from build123d import *

# Parameters (mm, degrees)
SKETCH1_W           = 160
SKETCH1_H           = 160
BOSS_EXTRUDE1_DEPTH = 18
SKETCH3_R           = 2
CUT_EXTRUDE1_DEPTH  = 115.560027933
SKETCH4_W           = 10
SKETCH4_H           = 18
BOSS_EXTRUDE3_DEPTH = 160
SKETCH7_R           = 2.75
CUT_EXTRUDE4_DEPTH  = 122.753850042


with BuildPart() as part:
    # Sketch1 → Boss-Extrude1 (new body)
    with BuildSketch(Plane.XY):
        Rectangle(SKETCH1_W, SKETCH1_H)
    extrude(amount=-BOSS_EXTRUDE1_DEPTH)

    # Sketch3 → Cut-Extrude1 (cut, through all)
    with BuildSketch(Plane.XY):
        with Locations((-76.5, 67.5)):
            Circle(SKETCH3_R)
        with Locations((-56.5, 67.5)):
            Circle(SKETCH3_R)
        with Locations((-56.5, 47.5)):
            Circle(SKETCH3_R)
        with Locations((-76.5, 47.5)):
            Circle(SKETCH3_R)
        with Locations((76.5, 67.5)):
            Circle(SKETCH3_R)
        with Locations((76.5, 47.5)):
            Circle(SKETCH3_R)
        with Locations((76.5, -47.5)):
            Circle(SKETCH3_R)
        with Locations((76.5, -67.5)):
            Circle(SKETCH3_R)
        with Locations((56.5, -47.5)):
            Circle(SKETCH3_R)
        with Locations((56.5, -67.5)):
            Circle(SKETCH3_R)
        with Locations((-56.5, -47.5)):
            Circle(SKETCH3_R)
        with Locations((-56.5, -67.5)):
            Circle(SKETCH3_R)
        with Locations((-76.5, -47.5)):
            Circle(SKETCH3_R)
        with Locations((-76.5, -67.5)):
            Circle(SKETCH3_R)
        with Locations((56.5, 67.5)):
            Circle(SKETCH3_R)
        with Locations((56.5, 47.5)):
            Circle(SKETCH3_R)
    extrude(amount=-CUT_EXTRUDE1_DEPTH, mode=Mode.SUBTRACT)

    # Sketch4 → Boss-Extrude3 (add)
    with BuildSketch(Plane(origin=(0, 80, 0), x_dir=(1, 0, 0), z_dir=(0, 1, 0))):
        with Locations((85, 9)):
            Rectangle(SKETCH4_W, SKETCH4_H)
        with Locations((-85, 9)):
            Rectangle(SKETCH4_W, SKETCH4_H)
    extrude(amount=-BOSS_EXTRUDE3_DEPTH)

    # Sketch7 → Cut-Extrude4 (cut, through all)
    with BuildSketch(Plane(origin=(0, 0, -18), x_dir=(-1, 0, 0), z_dir=(0, 0, -1))):
        with Locations((-20, -8)):
            Circle(SKETCH7_R)
        with Locations(Location((-20, -32, 0), (0, 0, 180))):
            Circle(SKETCH7_R)
        with Locations((20, -32)):
            Circle(SKETCH7_R)
        with Locations(Location((20, -8, 0), (0, 0, 180))):
            Circle(SKETCH7_R)
    extrude(amount=-CUT_EXTRUDE4_DEPTH, mode=Mode.SUBTRACT)


solid = part.part
Could you check a few things on this model? Use its own coordinates, in mm. Give positions to 0.01 mm unless a question says otherwise; leave off trailing zeros. Order: outer loops, then holes, each group sorted by start corner. A loop starts at its lowest first (then second) coordinate and runs counter-clockwise, first axis right, second up.
Item 1: If we mould it in two halves opening along Y, with no side actions, what happens to faces 1 (the face through (-1, -80, -9)), 2 (the face through (90, 1, -9)), 3 (the face through (-56.934, -49.452, -8.874)), 4 (the face through (-1, 80, -9))? For each: pulls with the +Y half, pulls with the -Y half, needs draft (parallel to the pull), parting line crosses it, or undercut.
Item 2: If we section it at A-A, the plane y = -8: Write out the boundary of the cut face in (x, z).
Item 3: If we section it at C-C, the plane x = 56.5: Write out the boundary of the cut face in (y, z), plus the area to 3 significant figures.
Item 4: If we section it at D-D, the plane y = 67.5: Write out the boundary of the cut face in (x, z).
Item 5: I need wall thicknesses on line 1 (Y direction, x = -76.5, z = -12.5); line 2 (Y direction, x = 56, z = -14.5); line 3 (X direction, y = -33.5, z = -16). Which ranges of each line are inside material? Lowest first, please.
Item 6: I'm going to push a flat-ended pin straight in: pin 1 (3 mm diameter, centred on x = -56.5, y = 47.5, fed in from -Z). Where does the tip first touch, or does it pass through?
Item 7: If we section it at B-B, the plane x = -20: Write out the boundary of the cut face in (y, z).
Values:
1. face 1: pulls with the -Y half
1. face 2: needs draft
1. face 3: undercut
1. face 4: pulls with the +Y half
2. outline: (-90, -18) - (-22.75, -18) - (-22.75, 0) - (-90, 0) - close; (-17.25, -18) - (17.25, -18) - (17.25, 0) - (-17.25, 0) - close; (22.75, -18) - (90, -18) - (90, 0) - (22.75, 0) - close
3. outline: (-80, -18) - (-69.5, -18) - (-69.5, 0) - (-80, 0) - close; (-65.5, -18) - (-49.5, -18) - (-49.5, 0) - (-65.5, 0) - close; (-45.5, -18) - (45.5, -18) - (45.5, 0) - (-45.5, 0) - close; (49.5, -18) - (65.5, -18) - (65.5, 0) - (49.5, 0) - close; (69.5, -18) - (80, -18) - (80, 0) - (69.5, 0) - close
3. area: 2,590 mm2
4. outline: (-90, -18) - (-78.5, -18) - (-78.5, 0) - (-90, 0) - close; (-74.5, -18) - (-58.5, -18) - (-58.5, 0) - (-74.5, 0) - close; (-54.5, -18) - (54.5, -18) - (54.5, 0) - (-54.5, 0) - close; (58.5, -18) - (74.5, -18) - (74.5, 0) - (58.5, 0) - close; (78.5, -18) - (90, -18) - (90, 0) - (78.5, 0) - close
5. line 1: y = -80 to -69.5, -65.5 to -49.5, -45.5 to 45.5, 49.5 to 65.5, 69.5 to 80
5. line 2: y = -80 to -69.44, -65.56 to -49.44, -45.56 to 45.56, 49.44 to 65.56, 69.44 to 80
5. line 3: x = -90 to -22.3, -17.7 to 17.7, 22.3 to 90
6. pin 1: passes through
7. outline: (-80, -18) - (-34.75, -18) - (-34.75, 0) - (-80, 0) - close; (-29.25, -18) - (-10.75, -18) - (-10.75, 0) - (-29.25, 0) - close; (-5.25, -18) - (80, -18) - (80, 0) - (-5.25, 0) - close
